The figure shows three views and two pictorial views of one solid part (mm, origin at its lowest corner). Answer the questions. Coordinates: 2 decimals unless noted, no trailing zeros. Write each loop counter-clockwise with the first axis right and the second up, starting at its lowest first coordinate (ties: lowest second). Pieces come first, ordered by that corner, then holes. Notation, with made-up numbers: M -30.5,-29.75 L 5.5,-29.75 A22 cw 5.5,-23.75 Z; hole C 13.5,-19 d6. An arc over 180 degrees is marked long. Write item = value, one per line.
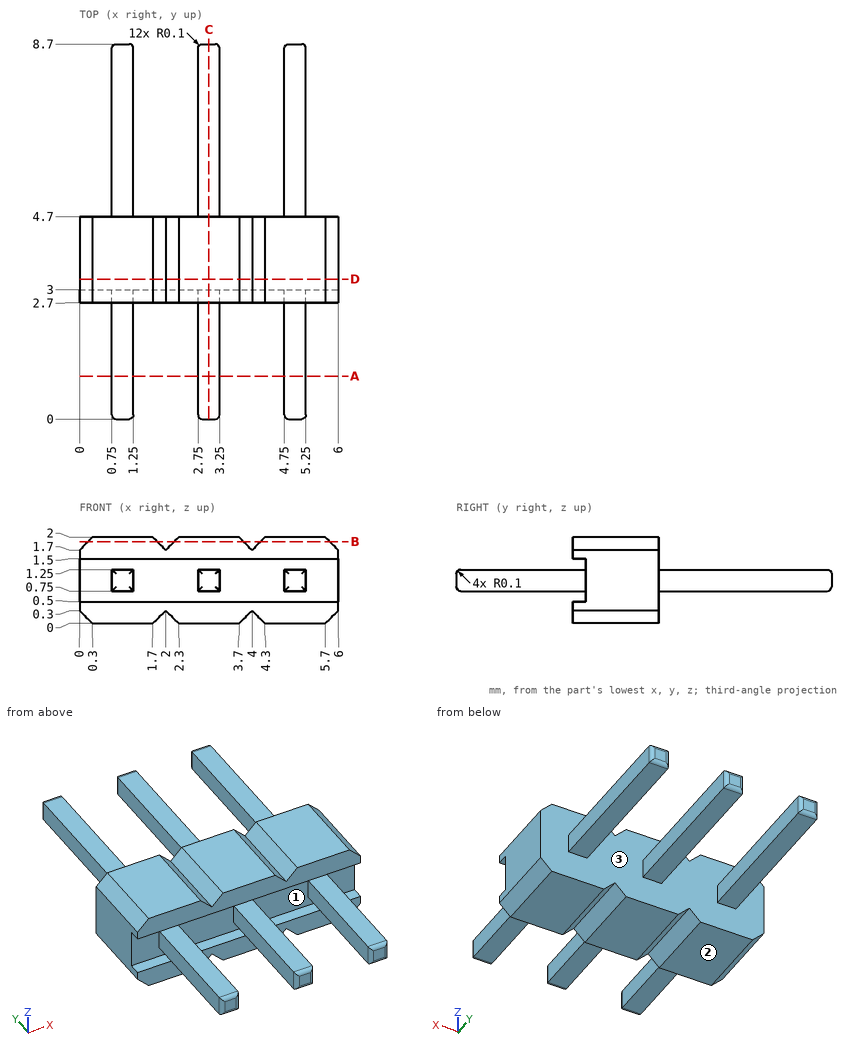
Item 1: Find section D-D (y = 3.25). Determine the outline of the cut face in (x, z).
Worked answers:
outline = M 0,0.3 L 0.3,0 L 1.7,0 L 2,0.3 L 2.3,0 L 3.7,0 L 4,0.3 L 4.3,0 L 5.7,0 L 6,0.3 L 6,1.7 L 5.7,2 L 4.3,2 L 4,1.7 L 3.7,2 L 2.3,2 L 2,1.7 L 1.7,2 L 0.3,2 L 0,1.7 Z
Item 2: Find section B-B (z = 1.9). Determine the outline of the cut face in (x, y), and give its area (3 significant figures).
Worked answers:
outline = M 0.2,2.7 L 1.8,2.7 L 1.8,4.7 L 0.2,4.7 Z; M 2.2,2.7 L 3.8,2.7 L 3.8,4.7 L 2.2,4.7 Z; M 4.2,2.7 L 5.8,2.7 L 5.8,4.7 L 4.2,4.7 Z
area = 9.60 mm²
Item 3: For a pull along Z with two mould halves and no side action, classify the marked faces 1, 2 and 3 as released by +Z, released by -Z, zero draft, split by the parting line, or undercut.
Worked answers:
face_1 = undercut
face_2 = released by -Z
face_3 = zero draft
Item 4: Consider line 1 along X through (y, z) = (1.75, 0.9); line 2 along X through (y, z) = (4.25, 1.8); line 3 along Y through (x, z) = (1.3, 1.65). Determine where each line is inside the solid, lowest interval first. Write a range as from..to.
Worked answers:
line_1 = 0.75..1.25, 2.75..3.25, 4.75..5.25
line_2 = 0.1..1.9, 2.1..3.9, 4.1..5.9
line_3 = 2.7..4.7
Item 5: Find section C-C (x = 3). Determine the outline of the cut face in (y, z), and give its area (3 significant figures).
Worked answers:
outline = M 0,0.85 A0.1 ccw 0.1,0.75 L 3,0.75 L 3,0.5 L 2.7,0.5 L 2.7,0 L 4.7,0 L 4.7,0.75 L 8.6,0.75 A0.1 ccw 8.7,0.85 L 8.7,1.15 A0.1 ccw 8.6,1.25 L 4.7,1.25 L 4.7,2 L 2.7,2 L 2.7,1.5 L 3,1.5 L 3,1.25 L 0.1,1.25 A0.1 ccw 0,1.15 Z
area = 7.19 mm²
Item 6: Flat-ended cylindrical pins translate along their axes: pin 1 (0.5 mm diameter, centred on x = 3, z = 1, fed in from -Y); pin 2 (0.6 mm diameter, centred on x = 5, y = 2, fed in from -Z); pin 3 (0.6 mm diameter, centred on x = 5, y = 5.5, fed in from +Z); pin 4 (1 mm diameter, centred on y = 5.5, z = 1.5, fed in from +X). Find the tip coordinate at first contact, or state that the pin passes through.
Worked answers:
pin_1 = 0
pin_2 = 0.75
pin_3 = 1.25
pin_4 = 5.25
Item 7: Find section A-A (y = 1). Determine the outline of the cut face in (x, z).
Worked answers:
outline = M 0.75,0.75 L 1.25,0.75 L 1.25,1.25 L 0.75,1.25 Z; M 2.75,0.75 L 3.25,0.75 L 3.25,1.25 L 2.75,1.25 Z; M 4.75,0.75 L 5.25,0.75 L 5.25,1.25 L 4.75,1.25 Z
